For this review, take the finished solid that the model builds, in its own axes (mm). A direction names the side the tool comes from. Round coordinates to 2 decimals unless told otherwise and drop trailing zeros. Order: outer loops, then holes, each group sorted by start corner. A loop starts at its lowest first (then second) coordinate and runs counter-clockwise, first axis right, second up. Notation, with made-up numbers: M 86.25,65.5 L 97.25,65.5 A8 ccw 97.25,77.5 Z; hole C 89.25,-27 d7. An arc over 180 degrees is marked long. Answer in a Markdown table with one row per item. Add a question column.
```python
from build123d import *

# Parameters (mm, degrees)
CROQUIS1_R              = 41
CROQUIS1_R_2            = 37.1125
SALIENTE_EXTRUIR1_DEPTH = 10
CROQUIS2_R              = 41
SALIENTE_EXTRUIR2_DEPTH = 10
CROQUIS3_R              = 29.25
CROQUIS3_R_2            = 23.25
CORTAR_EXTRUIR3_DEPTH   = 5
CROQUIS6_R              = 41
SALIENTE_EXTRUIR4_DEPTH = 5
CROQUIS8_R              = 41
CROQUIS8_R_2            = 34.6125
SALIENTE_EXTRUIR9_DEPTH = 2
CROQUIS10_W             = 40.5
CROQUIS10_H             = 20
CORTAR_EXTRUIR5_DEPTH   = 25
CROQUIS11_R             = 41
CROQUIS11_R_2           = 34.6125
CORTAR_EXTRUIR7_DEPTH   = 2
CROQUIS16_R             = 37.1125
CROQUIS16_R_2           = 29.25
CROQUIS16_R_3           = 23.25
CROQUIS16_R_4           = 0.131738941
CORTAR_EXTRUIR8_DEPTH   = 5
CORTAR_EXTRUIR11_DEPTH  = 13


with BuildPart() as part:
    # Croquis1 → Saliente-Extruir1 (new body)
    with BuildSketch(Plane(origin=(0, 0, 0), x_dir=(0, 0, -1), z_dir=(1, 0, 0))):
        Circle(CROQUIS1_R)
        Circle(CROQUIS1_R_2, mode=Mode.SUBTRACT)
    extrude(amount=SALIENTE_EXTRUIR1_DEPTH)

    # Croquis2 → Saliente-Extruir2 (add)
    with BuildSketch(Plane.ZY):
        Circle(CROQUIS2_R)
    extrude(amount=SALIENTE_EXTRUIR2_DEPTH)

    # Croquis3 → Cortar-Extruir3 (cut)
    with BuildSketch(Plane(origin=(0, 0, 0), x_dir=(0, 0, -1), z_dir=(1, 0, 0))):
        Circle(CROQUIS3_R)
        Circle(CROQUIS3_R_2, mode=Mode.SUBTRACT)
    extrude(amount=-CORTAR_EXTRUIR3_DEPTH, mode=Mode.SUBTRACT)

    # Croquis6 → Saliente-Extruir4 (add)
    with BuildSketch(Plane.ZY.offset(10)):
        Circle(CROQUIS6_R)
    extrude(amount=SALIENTE_EXTRUIR4_DEPTH)

    # Croquis8 → Saliente-Extruir9 (add)
    with BuildSketch(Plane(origin=(10, 0, 0), x_dir=(0, 0, -1), z_dir=(1, 0, 0))):
        Circle(CROQUIS8_R)
        Circle(CROQUIS8_R_2, mode=Mode.SUBTRACT)
    extrude(amount=-SALIENTE_EXTRUIR9_DEPTH)

    # Croquis10 → Cortar-Extruir5 (cut)
    with BuildSketch(Plane.ZY.offset(15)):
        with Locations((10.108898944, 0)):
            Rectangle(CROQUIS10_W, CROQUIS10_H)
    extrude(amount=-CORTAR_EXTRUIR5_DEPTH, mode=Mode.SUBTRACT)

    # Croquis11 → Cortar-Extruir7 (cut)
    with BuildSketch(Plane(origin=(10, 0, 0), x_dir=(0, 0, -1), z_dir=(1, 0, 0))):
        Circle(CROQUIS11_R)
        Circle(CROQUIS11_R_2, mode=Mode.SUBTRACT)
    extrude(amount=-CORTAR_EXTRUIR7_DEPTH, mode=Mode.SUBTRACT)

    # Croquis16 → Cortar-Extruir8 (cut)
    with BuildSketch(Plane(origin=(0, 0, 0), x_dir=(0, 0, -1), z_dir=(1, 0, 0))):
        Circle(CROQUIS16_R)
        Circle(CROQUIS16_R_2, mode=Mode.SUBTRACT)
        Circle(CROQUIS16_R_3)
        with Locations((-25.248825272, -14.504135598)):
            Circle(CROQUIS16_R_4)
    extrude(amount=-CORTAR_EXTRUIR8_DEPTH, mode=Mode.SUBTRACT)

    # Croquis17 → Cortar-Extruir11 (cut)
    with BuildSketch(Plane(origin=(8, 0, 0), x_dir=(0, 0, -1), z_dir=(1, 0, 0))):
        with BuildLine():
            Line((-52.12049427, 3.696100056), (-40.002976192, -8.986762253))
            ThreePointArc((-40.002976192, -8.986762253), (-40.999999439, 0.006784093), (-40, 9))
            Line((-40, 9), (-52.12049427, 3.696100056))
        make_face()
        with BuildLine():
            ThreePointArc((-36.004689365, 9), (-37.1125, 0), (-36.004689365, -9))
            Line((-36.004689365, -9), (-30.358898944, -9))
            Line((-30.358898944, -9), (-30.358898944, 9))
            Line((-30.358898944, 9), (-36.004689365, 9))
        make_face()
        with BuildLine():
            Line((-30.358898944, -9), (-36.004689365, -9))
            ThreePointArc((-36.004689365, -9), (4.533961965, -36.834506175), (37.1125, 0))
            ThreePointArc((37.1125, 0), (4.533961965, 36.834506175), (-36.004689365, 9))
            Line((-36.004689365, 9), (-30.358898944, 9))
            Line((-30.358898944, 9), (-30.358898944, -9))
        make_face()
        with BuildLine():
            Line((-40.002976192, -8.986762253), (-39.990328523, -9))
            Line((-39.990328523, -9), (-36.004689365, -9))
            ThreePointArc((-36.004689365, -9), (-37.1125, 0), (-36.004689365, 9))
            Line((-36.004689365, 9), (-40, 9))
            ThreePointArc((-40, 9), (-40.999999439, 0.006784093), (-40.002976192, -8.986762253))
        make_face()
    extrude(amount=-CORTAR_EXTRUIR11_DEPTH, mode=Mode.SUBTRACT)


solid = part.part
```
1. To check wall thickness, follow probe 1 along Y at (x, z) = (-2.5, -0.5); probe 2 along X at (y, z) = (29.5, 20); probe 3 along Z at (x, y) = (5, 0). State the ranges of each line that lie inside material, in increasing order. Write a range as [from, to].
2. The part is to be moulded in two halves that separate along Y. For faces 5 (the cylindrical face through (1.409, -1.505, -37.082)), 6 (the flat face through (8, -8.9, -36.3)), 7 (the flat face through (-10, 0, 30.359)), say which applies: pulls with the +Y half, pulls with the -Y half, needs draft (parallel to the pull), parting line crosses it, or undercut.
3. Consider section C-C on y = -25. Write out the cut boundary in (x, z), plus the area to 3 significant figures.
4. Consider section B-B on x = -11.25. Write out the cut boundary in (y, z).
5. For faces 1 (the flat face through (-5, 1, -15)), 2 (the flat face through (-10, 0, -10.141)), 3 (the flat face through (-15, -18, -1)), 4 (the flat face through (2, 9, 38)), list the 3-axis set-ups (+Z, -Z, +X, -X, +Y, -Y) from which the entire face can be reached by the end or side of a thin tool; tool diameter is ignored.
6. Clearance check with flat-ended pins moving along their axes: pin 1 Ø4 at (x, y) = (-12.5, 20) entering from +Z; pin 2 Ø2 at (x, z) = (3, 8.5) entering from +Y; pin 3 Ø12 at (x, y) = (-8.5, -7) entering from -Z; pin 4 Ø11 at (x, y) = (-12, -2.5) entering from +Z. State where each tip first meets the part, or that it passes through.
7. Consider section A-A on z = 0. Write out the cut boundary in (x, y), plus the area to 3 significant figures.
Solved:
| question | item | result |
|---|---|---|
| 1 | probe 1 | y = [-41, -37.11], [37.11, 41] |
| 1 | probe 2 | x = [-15, -5] |
| 1 | probe 3 | z = [-41, -37.11] |
| 2 | face 5 | undercut |
| 2 | face 6 | needs draft |
| 2 | face 7 | undercut |
| 3 | outline | M -15,-32.5 L 8,-32.5 L 8,-27.43 L -5,-27.43 L -5,27.43 L 8,27.43 L 8,32.5 L -15,32.5 Z |
| 3 | area | 782 mm^2 |
| 4 | outline | C 0,0 d82; hole M -10,-10.14 L 10,-10.14 L 10,30.36 L -10,30.36 Z |
| 5 | face 1 | +X |
| 5 | face 2 | +X, -X |
| 5 | face 3 | +Z, -Z, -X, +Y, -Y |
| 5 | face 4 | +Z, +X |
| 6 | pin 1 | stops at z = 36.84 |
| 6 | pin 2 | stops at y = 40.31 |
| 6 | pin 3 | stops at z = -40.99 |
| 6 | pin 4 | stops at z = 41 |
| 7 | outline | M -15,-41 L 8,-41 L 8,-37.11 L -5,-37.11 L -5,-10 L -15,-10 Z; M -15,10 L -5,10 L -5,37.11 L 8,37.11 L 8,41 L -15,41 Z |
| 7 | area | 721 mm^2 |
